```python
from build123d import *

# Parameters (mm, degrees)
BOSS_EXTRUDE1_DEPTH = 9
SKETCH2_R           = 2.75
CUT_EXTRUDE1_DEPTH  = 4
SKETCH3_R           = 2.75
CUT_EXTRUDE2_DEPTH  = 4


with BuildPart() as part:
    # Sketch1 → Boss-Extrude1 (new body, symmetric)
    with BuildSketch(Plane.XY):
        with BuildLine():
            Line((0, 0), (0, 40))
            Line((0, 40), (3, 40))
            Line((3, 40), (3, 4))
            ThreePointArc((3, 4), (3.292893219, 3.292893219), (4, 3))
            Line((4, 3), (40, 3))
            Line((40, 3), (40, 0))
            Line((40, 0), (0, 0))
        make_face()
    extrude(amount=BOSS_EXTRUDE1_DEPTH, both=True)

    # Sketch2 → Cut-Extrude1 (cut, through all)
    with BuildSketch(Plane(origin=(3, 0, 0), x_dir=(0, 0, -1), z_dir=(1, 0, 0))):
        with Locations((0, 10)):
            Circle(SKETCH2_R)
        with Locations((0, 30)):
            Circle(SKETCH2_R)
    extrude(amount=-CUT_EXTRUDE1_DEPTH, mode=Mode.SUBTRACT)

    # Sketch3 → Cut-Extrude2 (cut, through all)
    with BuildSketch(Plane(origin=(0, 3, 0), x_dir=(1, 0, 0), z_dir=(0, 1, 0))):
        with Locations((10, 0)):
            Circle(SKETCH3_R)
        with Locations((30, 0)):
            Circle(SKETCH3_R)
    extrude(amount=-CUT_EXTRUDE2_DEPTH, mode=Mode.SUBTRACT)


solid = part.part
```
The listing builds one solid part. Answer for the finished solid, in the listing's coordinates (mm). A direction names the side the tool comes from. Give positions to 0.01 mm unless a question says otherwise; leave off trailing zeros. Order: outer loops, then holes, each group sorted by start corner. A loop starts at its lowest first (then second) coordinate and runs counter-clockwise, first axis right, second up.
1) Find section D-D on z = -7.5. Write down the section's boundary in (x, y).
Reported:
outline: (0, 0) - (40, 0) - (40, 3) - (4, 3) arc R1 cw to (3, 4) - (3, 40) - (0, 40) - close
2) For faces 5 (the face through (40, 2, 0)), 6 (the face through (22, 3, 0)), determine the directions among +Z, -Z, +X, -X, +Y, -Y from which every point of the face is accessible in a straight line to the end or side of a thin tool.
Reported:
face 5: +Z, -Z, +X, +Y, -Y
face 6: +Z, -Z, +X, +Y
3) Given P1, Ø4.5, axis at y = 10, z = 0, coming from the +X side; P2, Ø8, axis at x = 31, z = 6.5, coming from the +Y side; P3, Ø1.5, axis at y = 6.5, z = 3.5, coming from the +X side, each flat-ended and moving along its own axis, determine where each tip first touches the part or whether it passes through.
Reported:
P1: passes through
P2: stops at y = 3
P3: stops at x = 3
4) Consider line 1 along X through (y, z) = (2.2, 0); line 2 along Z through (x, y) = (10, 2.3). Determine where each line is inside the solid, lowest interval first.
Reported:
line 1: x = 0 to 7.25, 12.75 to 27.25, 32.75 to 40
line 2: z = -9 to -2.75, 2.75 to 9
5) Find section B-B on x = 10. Write down the section's boundary in (y, z).
Reported:
outline: (0, -9) - (3, -9) - (3, -2.75) - (0, -2.75) - close; (0, 2.75) - (3, 2.75) - (3, 9) - (0, 9) - close
6) Determine the mould class of faces 1 (the face through (11, 2, 9)), 2 (the face through (11, 2, -9)), 3 (the face through (1.521, 32.727, 0.358)), 4 (the face through (20, 0, 0)) for opening direction Z: pulls with the +Z half, pulls with the -Z half, needs draft (parallel to the pull), parting line crosses it, or undercut.
Reported:
face 1: pulls with the +Z half
face 2: pulls with the -Z half
face 3: undercut
face 4: needs draft
7) Find section A-A on z = 0. Write down the section's boundary in (x, y).
Reported:
outline: (0, 0) - (7.25, 0) - (7.25, 3) - (4, 3) arc R1 cw to (3, 4) - (3, 7.25) - (0, 7.25) - close; (0, 12.75) - (3, 12.75) - (3, 27.25) - (0, 27.25) - close; (0, 32.75) - (3, 32.75) - (3, 40) - (0, 40) - close; (12.75, 0) - (27.25, 0) - (27.25, 3) - (12.75, 3) - close; (32.75, 0) - (40, 0) - (40, 3) - (32.75, 3) - close
